Here's how the part is built. I have some questions about the finished solid (model axes, mm). Round coordinates to 2 decimals unless told otherwise and drop trailing zeros. Order: outer loops, then holes, each group sorted by start corner. A loop starts at its lowest first (then second) coordinate and runs counter-clockwise, first axis right, second up.
```python
from build123d import *

# Parameters (mm, degrees)
BOSS_EXTRUDE2_DEPTH = 5
SKETCH2_R           = 10.345071301
CUT_EXTRUDE1_DEPTH  = 5
SKETCH3_R           = 11.936620732
CUT_EXTRUDE2_DEPTH  = 5
SKETCH5_R           = 12.732395447
CUT_EXTRUDE3_DEPTH  = 5
SKETCH6_R           = 11.936620732
CUT_EXTRUDE4_DEPTH  = 5


with BuildPart() as part:
    # Sketch1 → Boss-Extrude2 (new body)
    with BuildSketch(Plane.XY):
        with BuildLine():
            ThreePointArc((-10.756876138, -13.082000519), (2.738805764, -16.713708888), (14.369566376, -8.964635184))
            ThreePointArc((14.369566376, -8.964635184), (26.589818025, -17.463000516), (40.979710452, -13.656721546))
            ThreePointArc((40.979710452, -13.656721546), (73.463989272, -15.940066616), (47.111882074, 3.191281517))
            ThreePointArc((47.111882074, 3.191281517), (32.748214335, 17.463000516), (14.369566376, 8.964635184))
            ThreePointArc((14.369566376, 8.964635184), (-3.142789543, 16.642475648), (-16.649193034, 3.107007102))
            ThreePointArc((-16.649193034, 3.107007102), (-40.05605495, -14.579211704), (-10.756876138, -13.082000519))
        make_face()
    extrude(amount=BOSS_EXTRUDE2_DEPTH)

    # Sketch2 → Cut-Extrude1 (cut)
    with BuildSketch(Plane.XY.offset(5)):
        with Locations((-25.636404683, -9.330888218)):
            Circle(SKETCH2_R)
    extrude(amount=-CUT_EXTRUDE1_DEPTH, mode=Mode.SUBTRACT)

    # Sketch3 → Cut-Extrude2 (cut)
    with BuildSketch(Plane.XY.offset(5)):
        Circle(SKETCH3_R)
    extrude(amount=-CUT_EXTRUDE2_DEPTH, mode=Mode.SUBTRACT)

    # Sketch5 → Cut-Extrude3 (cut)
    with BuildSketch(Plane.XY.offset(5)):
        with Locations((29.66901618, 0)):
            Circle(SKETCH5_R)
    extrude(amount=-CUT_EXTRUDE3_DEPTH, mode=Mode.SUBTRACT)

    # Sketch6 → Cut-Extrude4 (cut)
    with BuildSketch(Plane.XY.offset(5)):
        with Locations((57.54877175, -10.147401166)):
            Circle(SKETCH6_R)
    extrude(amount=-CUT_EXTRUDE4_DEPTH, mode=Mode.SUBTRACT)


solid = part.part
```
1) I'm going to push flat-ended pins straight in: pin 1 (1.5 mm diameter, centred on y = 0.5, z = 4, fed in from -X); pin 2 (14.5 mm diameter, centred on x = 0, y = 0, fed in from -Z); pin 3 (2 mm diameter, centred on x = -8, z = 2, fed in from +Y); pin 4 (1.5 mm diameter, centred on x = 47.5, z = 1.5, fed in from -Y). Where does each tip first touch, or does it pass through?
2) If we section it at B-B (y = 0): Write out the boundary of the cut face in (x, z), plus the area to 3 significant figures.
3) If we section it at A-A (x = 0): Write out the boundary of the cut face in (y, z).
4) We'd pull the mould along X, two halves only. Please class faces 1 (the cylindrical face through (33.04, 17.41, 2.46)), 2 (the flat face through (16, -5, 5)): +X half, -X half, draft (parallel to the pull), parting line (faces both ways), or undercut.
5) I need wall thicknesses on line 1 (Y direction, x = -25, z = 4.5); line 2 (Y direction, x = 0, z = 3.8); line 3 (X direction, y = -1.5, z = 4.3). Which ranges of each line are inside material? Lowest first, please.
6) If we section it at D-D (x = 27): Write out the boundary of the cut face in (y, z).
7) If we section it at C-C (z = 1.6): Write out the boundary of the cut face in (x, y).
Solutions:
1. pin 1: stops at x = -38.01
1. pin 2: passes through
1. pin 3: stops at y = 15.42
1. pin 4: stops at y = -24.3
2. outline: (-37.82, 0) - (-30.1, 0) - (-30.1, 5) - (-37.82, 5) - close; (-21.17, 0) - (-11.94, 0) - (-11.94, 5) - (-21.17, 5) - close; (11.94, 0) - (16.94, 0) - (16.94, 5) - (11.94, 5) - close; (42.4, 0) - (51.26, 0) - (51.26, 5) - (42.4, 5) - close; (63.83, 0) - (71.11, 0) - (71.11, 5) - (63.83, 5) - close
2. area: 190 mm2
3. outline: (-16.94, 0) - (-11.94, 0) - (-11.94, 5) - (-16.94, 5) - close; (11.94, 0) - (16.94, 0) - (16.94, 5) - (11.94, 5) - close
4. face 1: undercut
4. face 2: draft
5. line 1: y = -24.66 to -19.66, 0.99 to 6
5. line 2: y = -16.94 to -11.94, 11.94 to 16.94
5. line 3: x = -38.83 to -32.4, -18.88 to -11.84, 11.84 to 17.03, 42.31 to 49.32, 65.78 to 72.11
6. outline: (-17.53, 0) - (-12.45, 0) - (-12.45, 5) - (-17.53, 5) - close; (12.45, 0) - (17.53, 0) - (17.53, 5) - (12.45, 5) - close
7. outline: (-16.65, 3.11) arc R15.35 ccw (long way) to (-10.76, -13.08) arc R16.94 ccw to (14.37, -8.96) arc R17.73 ccw to (40.98, -13.66) arc R16.94 ccw (long way) to (47.11, 3.19) arc R17.73 ccw to (14.37, 8.96) arc R16.94 ccw to start; hole circle Ø20.69 at (-25.64, -9.33); hole circle Ø23.87 at (0, 0); hole circle Ø25.46 at (29.67, 0); hole circle Ø23.87 at (57.55, -10.15)
